Part model, mm, in its own coordinate system. A direction names the side the tool comes from. Give positions to 0.01 mm unless a question says otherwise; leave off trailing zeros. Order: outer loops, then holes, each group sorted by start corner. A loop starts at its lowest first (then second) coordinate and runs counter-clockwise, first axis right, second up.
from build123d import *

# Parameters (mm, degrees)
BOSS_EXTRUDE1_DEPTH = 8
BOSS_EXTRUDE2_DEPTH = 10
CUT_EXTRUDE1_REACH  = 20
SKETCH3_R           = 4
FILLET1_R           = 1
CUT_EXTRUDE3_DEPTH  = 4.5
FILLET2_R           = 2


with BuildPart() as part:
    # Sketch1 → Boss-Extrude1 (new body)
    with BuildSketch(Plane.XY):
        with BuildLine():
            Line((49.740147273, 55.788144293), (49.740147273, 48.788144293))
            Line((49.740147273, 48.788144293), (154.737534778, 48.788144293))
            Line((154.737534778, 48.788144293), (154.737534778, 55.264402854))
            ThreePointArc((154.737534778, 55.264402854), (102.50202125, 108.287491165), (49.740147273, 55.788144293))
        make_face()
    extrude(amount=BOSS_EXTRUDE1_DEPTH)

    # Sketch2 → Boss-Extrude2 (add)
    with BuildSketch(Plane.XY.offset(8)):
        with BuildLine():
            Line((159.740147273, 55.788144293), (159.740147273, 48.788144293))
            Line((159.740147273, 48.788144293), (44.740147273, 48.788144293))
            Line((44.740147273, 48.788144293), (44.740147273, 55.788144293))
            ThreePointArc((44.740147273, 55.788144293), (102.240147273, 113.288144293), (159.740147273, 55.788144293))
        make_face()
    extrude(amount=BOSS_EXTRUDE2_DEPTH)

    # Sketch3 → Cut-Extrude1 (cut, up to next)
    with BuildSketch(Plane.XY.offset(18), mode=Mode.PRIVATE) as cut_extrude1_sk1:
        with Locations((87.240147273, 55.788144293)):
            Circle(SKETCH3_R)
    cut_extrude1_tool1 = extrude(cut_extrude1_sk1.sketch, amount=-CUT_EXTRUDE1_REACH, mode=Mode.PRIVATE) & part.part
    add(cut_extrude1_tool1.solids().sort_by_distance((87.240147, 55.788144, 18))[0], mode=Mode.SUBTRACT)

    # Fillet1
    fillet1_edges = [part.edges().sort_by_distance(p)[0] for p in [
        (159.740147273, 52.288144293, 8),
        (44.740147273, 52.288144293, 8),
        (159.740147273, 52.288144293, 18),
        (44.740147273, 52.288144293, 18),
        (102.240147273, 113.288144293, 8),
        (102.240147273, 113.288144293, 18),
    ]]
    fillet(fillet1_edges, radius=FILLET1_R)

    # Sketch6 → Cut-Extrude3 (cut)
    with BuildSketch(Plane.XY):
        with BuildLine():
            Line((72.39178204, 48.788144293), (57.39178204, 48.788144293))
            Line((57.39178204, 48.788144293), (57.39178204, 58.754668066))
            ThreePointArc((57.39178204, 58.754668066), (64.89178204, 66.254668066), (72.39178204, 58.754668066))
            Line((72.39178204, 58.754668066), (72.39178204, 48.788144293))
        make_face()
    extrude(amount=CUT_EXTRUDE3_DEPTH, mode=Mode.SUBTRACT)

    # Fillet2
    fillet2_edges = [part.edges().sort_by_distance(p)[0] for p in [
        (64.89178204, 66.254668066, 0),
        (57.39178204, 53.771406179, 0),
        (72.39178204, 53.771406179, 0),
        (64.89178204, 66.254668066, 4.5),
        (57.39178204, 53.771406179, 4.5),
        (72.39178204, 53.771406179, 4.5),
    ]]
    fillet(fillet2_edges, radius=FILLET2_R)


solid = part.part
Item 1: Drill centre lines: probe 1 along Z at (x, y) = (90, 109.5); probe 2 along Y at (x, z) = (63.5, 7); probe 3 along X at (y, z) = (80.5, 17.25). Where is each one in solid material? Low to high.
Item 2: Drop flat-ended pins along their axis: P1, Ø7.5, axis at y = 53, z = 2.5, coming from the -X side; P2, Ø12, axis at x = 67, y = 53, coming from the -Z side; P3, Ø10, axis at x = 138, z = 13, coming from the +Y side. Give the stop position or say it passes through.
Item 3: Which spindle directions (+Z, -Z, +X, -X, +Y, -Y) get a long thin tool onto all of the face, cutting with end or side? Do faces 1 (the face through (154.738, 52, 4)), 2 (the face through (102, 72, 0)), 3 (the face through (57.993, 53.841, 3.93)). Say none if no direction does.
Item 4: Band-saw the part on A-A on z = 15.5. List the corners of the cut face in (x, y).
Item 5: Pull direction X, two halves, no side cores. Call faces 4 (the face through (56.79, 53.84, 0.57)), 5 (the face through (49.74, 52, 4)), 6 (the face through (65, 57, 4.5)), 7 (the face through (103, 109, 8)): released by +X, released by -X, zero draft, split by the parting line, or undercut.
Working result:
1. probe 1: z = 8 to 18
1. probe 2: y = 48.79 to 91.22
1. probe 3: x = 50.36 to 154.12
2. P1: stops at x = 49.74
2. P2: stops at z = 0.56
2. P3: stops at y = 104.37
3. face 1: -Z, +X, +Y, -Y
3. face 2: -Z, +X, -X, +Y, -Y
3. face 3: -Z, -Y
4. outline: (44.74, 48.79) - (159.74, 48.79) - (159.74, 55.79) arc R57.5 ccw to (44.74, 55.79) - close; hole circle Ø8 at (87.24, 55.79)
5. face 4: undercut
5. face 5: released by -X
5. face 6: undercut
5. face 7: zero draft
